Check sheet for the drawn part. Datum: minimum x, y, z corner. Units: mm. A direction names the side the tool comes from. Coordinates: 2 decimals unless noted, no trailing zeros. Write each loop counter-clockwise with the first axis right and the second up, starting at its lowest first coordinate (ties: lowest second). Pieces come first, ordered by that corner, then holes. Notation, with made-up numbers: (8.5, 21) -> (63.5, 21) arc R15 cw to (63.5, 42) -> close; hole circle Ø2 at (-16.5, 62). An arc over 180 degrees is marked (long way). Answer in a Markdown table with one row per item. Add a question column.
Q1. Section check C-C, the plane x = 28.75. Record the boundary of the cut face in (y, z), and give its area (3 significant figures).
Q2. Section check D-D, the plane z = 5.5. Record the boundary of the cut face in (x, y) (3 decimals), and give its area (3 significant figures).
Q3. Tool access check on the marked faces 1 and 2. Record the directions out of +Z, -Z, +X, -X, +Y, -Y that give a thin tool (end or side, any length) a straight path to the whole face; none if there is none.
Q4. Release check for a two-part mould opening along X. For the marked faces 3, 4 and 5 record: pulls with the +X half, pulls with the -X half, needs draft (parallel to the pull), parting line crosses it, or undercut.
Q5. Thickness scan on line 1 (X direction, y = 5.6, z = 19.66); line 2 (Z direction, x = 5.5, y = 4.6); line 3 (X direction, y = 2.9, z = 3.5). Record the ranges inside material, lowest first.
Q6. Gauge pin test, flat ends, axial feed: P1, Ø9.5, axis at x = 10, z = 22.5, coming from the -Y side; P2, Ø1.2, axis at x = 16.5, y = 1.5, coming from the -Z side; P3, Ø2.5, axis at x = 17.125, z = 5.5, coming from the -Y side. Record the tip position at first contact, or that the pin passes through.
Q7. Section check B-B, the plane z = 19.66. Record the boundary of the cut face in (x, y), and give its area (3 significant figures).
Q8. Section check A-A, the plane y = 4.5. Record the boundary of the cut face in (x, z) (3 decimals).
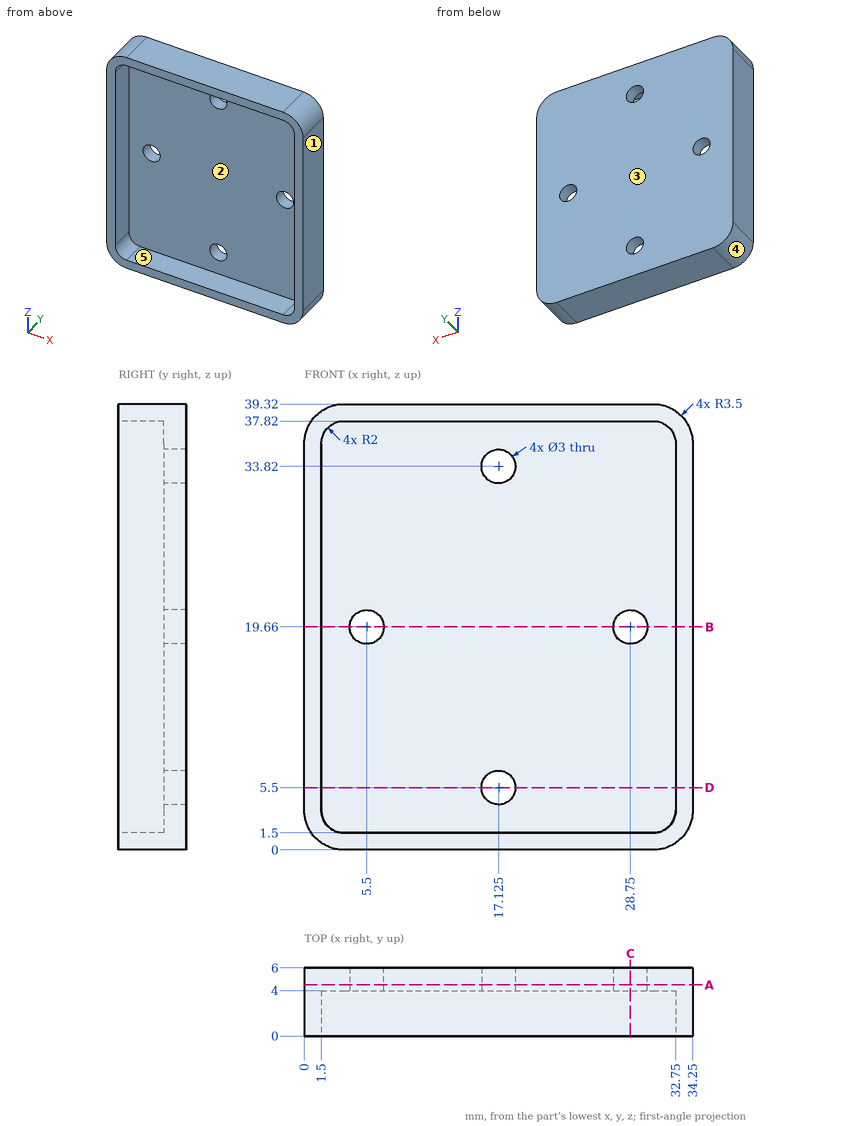
Calculated:
| question | item | result |
|---|---|---|
| 1 | outline | (0, 0) -> (6, 0) -> (6, 18.16) -> (4, 18.16) -> (4, 1.5) -> (0, 1.5) -> close; (0, 37.82) -> (4, 37.82) -> (4, 21.16) -> (6, 21.16) -> (6, 39.32) -> (0, 39.32) -> close |
| 1 | area | 84.6 mm² |
| 2 | outline | (0, 0) -> (1.5, 0) -> (1.5, 4) -> (15.625, 4) -> (15.625, 6) -> (0, 6) -> close; (18.625, 4) -> (32.75, 4) -> (32.75, 0) -> (34.25, 0) -> (34.25, 6) -> (18.625, 6) -> close |
| 2 | area | 74.5 mm² |
| 3 | face 1 | +Z, -Z, +X, +Y, -Y |
| 3 | face 2 | -Y |
| 4 | face 3 | needs draft |
| 4 | face 4 | pulls with the -X half |
| 4 | face 5 | undercut |
| 5 | line 1 | x = 0 to 4, 7 to 27.25, 30.25 to 34.25 |
| 5 | line 2 | z = 0 to 18.16, 21.16 to 39.32 |
| 5 | line 3 | x = 0 to 1.5, 32.75 to 34.25 |
| 6 | P1 | stops at y = 4 |
| 6 | P2 | stops at z = 0 |
| 6 | P3 | passes through |
| 7 | outline | (0, 0) -> (1.5, 0) -> (1.5, 4) -> (4, 4) -> (4, 6) -> (0, 6) -> close; (7, 4) -> (27.25, 4) -> (27.25, 6) -> (7, 6) -> close; (30.25, 4) -> (32.75, 4) -> (32.75, 0) -> (34.25, 0) -> (34.25, 6) -> (30.25, 6) -> close |
| 7 | area | 68.5 mm² |
| 8 | outline | (0, 3.5) arc R3.5 ccw to (3.5, 0) -> (30.75, 0) arc R3.5 ccw to (34.25, 3.5) -> (34.25, 35.82) arc R3.5 ccw to (30.75, 39.32) -> (3.5, 39.32) arc R3.5 ccw to (0, 35.82) -> close; hole circle Ø3 at (5.5, 19.66); hole circle Ø3 at (17.125, 5.5); hole circle Ø3 at (17.125, 33.82); hole circle Ø3 at (28.75, 19.66) |
